Read the model definition and answer for the solid it produces. Units are mm, in the model's axes. Give positions to 0.01 mm unless a question says otherwise; leave off trailing zeros. Order: outer loops, then holes, each group sorted by start corner. A loop starts at its lowest first (then second) coordinate and runs counter-clockwise, first axis right, second up. Notation, with made-up numbers: M 15,1.5 L 32,1.5 A34 ccw 32,37.5 Z; hole C 27.25,7.5 d4. An arc over 180 degrees is marked long. Write item = value, one per line. Start each with the question number.
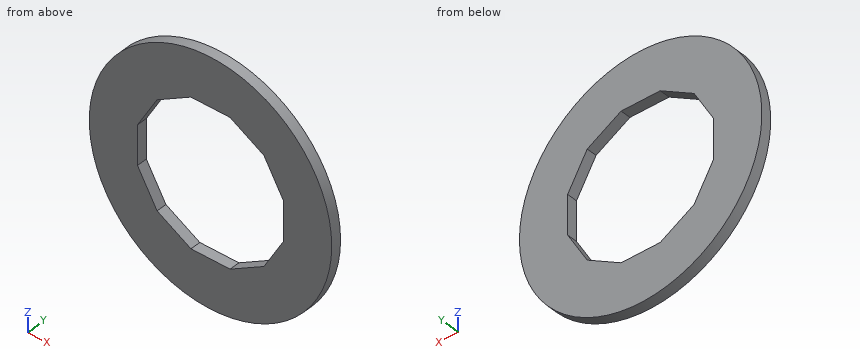
from build123d import *

# Parameters (mm, degrees)
F0_R     = 70
F1_DEPTH = 3


# Not quite as in the source:
# - a feature of the source that left no trace in its solid (it failed there, or was rolled back) is left out


with BuildPart() as f1:
    # F0 (on Front) → F1 (new body, symmetric)
    with BuildSketch(Plane.XZ):
        Circle(F0_R)
        Polygon((-30.855941539, 30.855941539), (-11.294058461, 42.15), (11.294058461, 42.15), (30.855941539, 30.855941539), (42.15, 11.294058461), (42.15, -11.294058461), (30.855941539, -30.855941539), (11.294058461, -42.15), (-11.294058461, -42.15), (-30.855941539, -30.855941539), (-42.15, -11.294058461), (-42.15, 11.294058461), align=None, mode=Mode.SUBTRACT)
    extrude(amount=F1_DEPTH, both=True)


solid = f1.part
1) Find section C-C on z = 0. Determine the outline of the cut face in (x, y), plus the area to 3 significant figures.
2) Find section B-B on y = -1.2. Determine the outline of the cut face in (x, z), plus the area to 3 significant figures.
3) Find section A-A on x = 0. Determine the outline of the cut face in (y, z), plus the area to 3 significant figures.
4) Find the intervals of material crossed by probe 1 along X at (y, z) = (-0.4, -0.5); probe 2 along Z at (x, y) = (-2.5, 2.05), in increasing order. Write a range as [from, to].
5) Each of these flat-tipped pins is pushed along its axis until it touches: P1, Ø2, axis at x = -37.5, y = -0.5, coming from the +Z side; P2, Ø3, axis at y = 0, z = 43, coming from the -X side; P3, Ø1.8, axis at y = 1, z = 3.5, coming from the +X side. Where does it stop, or does it pass through?
6) Find section D-D on z = 60. Determine the outline of the cut face in (x, y), plus the area to 3 significant figures.
Numbers:
q1.outline = M -70,-3 L -42.15,-3 L -42.15,3 L -70,3 Z; M 42.15,-3 L 70,-3 L 70,3 L 42.15,3 Z
q1.area = 334 mm2
q2.outline = C 0,0 d140; hole M -42.15,-11.29 L -30.86,-30.86 L -11.29,-42.15 L 11.29,-42.15 L 30.86,-30.86 L 42.15,-11.29 L 42.15,11.29 L 30.86,30.86 L 11.29,42.15 L -11.29,42.15 L -30.86,30.86 L -42.15,11.29 Z
q2.area = 9,680 mm2
q3.outline = M -3,-70 L 3,-70 L 3,-42.15 L -3,-42.15 Z; M -3,42.15 L 3,42.15 L 3,70 L -3,70 Z
q3.area = 334 mm2
q4.probe_1 = [-70, -42.15], [42.15, 70]
q4.probe_2 = [-69.96, -42.15], [42.15, 69.96]
q5.P1 = 59.73
q5.P2 = -56.37
q5.P3 = 69.95
q6.outline = M -36.06,-3 L 36.06,-3 L 36.06,3 L -36.06,3 Z
q6.area = 433 mm2
